Could you check a few things on this model? Use its own coordinates, in mm. A direction names the side the tool comes from. Give positions to 0.01 mm unless a question says otherwise; leave off trailing zeros. Loops run counter-clockwise (first coordinate to the right, second up) from the corner with the lowest first, then second, coordinate; pieces in that order, holes last. Notation, with made-up numbers: M 60,-40 L 83,-40 A17 ccw 83,-13 Z; hole C 69,16 d7. An arc over 180 degrees is marked long. Answer in a Markdown table with one row per item. Add a question column.
```python
from build123d import *

# Parameters (mm, degrees)
SKETCH1_W           = 15
SKETCH1_H           = 21.5
SKETCH1_W_2         = 21.5
SKETCH1_H_2         = 15
BOSS_EXTRUDE1_DEPTH = 1.5
BOSS_EXTRUDE2_START = -1.5
SKETCH2_W           = 1.5
SKETCH2_H           = 15
BOSS_EXTRUDE2_DEPTH = 28.5
BOSS_EXTRUDE3_START = -1.5
SKETCH3_W           = 15
SKETCH3_H           = 1.5
BOSS_EXTRUDE3_DEPTH = 28.5
SKETCH4_R           = 1.5
CUT_EXTRUDE1_DEPTH  = 62
SKETCH5_R           = 1.5
CUT_EXTRUDE2_DEPTH  = 62
FILLET1_R           = 2
FILLET2_R           = 2
FILLET3_R           = 18
CUT_EXTRUDE3_REACH  = 63
SKETCH6_R           = 4
CUT_EXTRUDE4_REACH  = 63
SKETCH7_R           = 4


with BuildPart() as part:
    # Sketch1 → Boss-Extrude1 (new body)
    with BuildSketch(Plane.XY):
        with Locations((0, 18.25)):
            Rectangle(SKETCH1_W, SKETCH1_H)
        with Locations((-18.25, 0)):
            Rectangle(SKETCH1_W_2, SKETCH1_H_2)
        Rectangle(SKETCH1_W, SKETCH1_H_2)
        with Locations((18.25, 0)):
            Rectangle(SKETCH1_W_2, SKETCH1_H_2)
        with Locations((0, -18.25)):
            Rectangle(SKETCH1_W, SKETCH1_H)
    extrude(amount=BOSS_EXTRUDE1_DEPTH)

    # Sketch2 → Boss-Extrude2 (add)
    with BuildSketch(Plane.XY.offset(1.5).offset(BOSS_EXTRUDE2_START)):
        with Locations((-29.75, 0)):
            Rectangle(SKETCH2_W, SKETCH2_H)
        with Locations((29.75, 0)):
            Rectangle(SKETCH2_W, SKETCH2_H)
    extrude(amount=BOSS_EXTRUDE2_DEPTH)

    # Sketch3 → Boss-Extrude3 (add)
    with BuildSketch(Plane(origin=(0, 0, 0), x_dir=(-1, 0, 0), z_dir=(0, 0, -1)).offset(BOSS_EXTRUDE3_START)):
        with Locations((0, 29.75)):
            Rectangle(SKETCH3_W, SKETCH3_H)
        with Locations((0, -29.75)):
            Rectangle(SKETCH3_W, SKETCH3_H)
    extrude(amount=BOSS_EXTRUDE3_DEPTH)

    # Sketch4 → Cut-Extrude1 (cut, through all)
    with BuildSketch(Plane(origin=(30.5, 0, 0), x_dir=(0, 0, -1), z_dir=(1, 0, 0))):
        with Locations((-22.5, 0)):
            Circle(SKETCH4_R)
    extrude(amount=-CUT_EXTRUDE1_DEPTH, mode=Mode.SUBTRACT)

    # Sketch5 → Cut-Extrude2 (cut, through all)
    with BuildSketch(Plane(origin=(0, 30.5, 0), x_dir=(1, 0, 0), z_dir=(0, 1, 0))):
        with Locations((0, 21)):
            Circle(SKETCH5_R)
    extrude(amount=-CUT_EXTRUDE2_DEPTH, mode=Mode.SUBTRACT)

    # Fillet1
    fillet1_edges = [part.edges().sort_by_distance(p)[0] for p in [
        (-7.5, -29.75, -27),
        (7.5, -29.75, -27),
        (-7.5, 29.75, -27),
        (7.5, 29.75, -27),
        (-29.75, 7.5, 28.5),
        (-29.75, -7.5, 28.5),
        (29.75, -7.5, 28.5),
        (29.75, 7.5, 28.5),
    ]]
    fillet(fillet1_edges, radius=FILLET1_R)

    # Fillet2
    fillet2_edges = [part.edges().sort_by_distance(p)[0] for p in [
        (29, 0, 1.5),
        (30.5, 0, 0),
        (-30.5, 0, 0),
        (-29, 0, 1.5),
        (0, 29, 0),
        (0, -29, 0),
        (0, -30.5, 1.5),
        (0, 30.5, 1.5),
    ]]
    fillet(fillet2_edges, radius=FILLET2_R)

    # Fillet3
    fillet3_edges = [part.edges().sort_by_distance(p)[0] for p in [
        (-7.5, 7.5, 0.75),
        (-7.5, -7.5, 0.75),
        (7.5, -7.5, 0.75),
        (7.5, 7.5, 0.75),
    ]]
    fillet(fillet3_edges, radius=FILLET3_R)

    # Sketch6 → Cut-Extrude3 (cut, up to next)
    with BuildSketch(Plane(origin=(30.5, 0, 0), x_dir=(0, 0, -1), z_dir=(1, 0, 0)), mode=Mode.PRIVATE) as cut_extrude3_sk1:
        with Locations((-22.5, 0)):
            Circle(SKETCH6_R)
    cut_extrude3_tool1 = extrude(cut_extrude3_sk1.sketch, amount=-CUT_EXTRUDE3_REACH, mode=Mode.PRIVATE) & part.part
    add(cut_extrude3_tool1.solids().sort_by_distance((30.5, 0, 22.5))[0], mode=Mode.SUBTRACT)

    # Sketch7 → Cut-Extrude4 (cut, up to next)
    with BuildSketch(Plane.XZ.offset(30.5), mode=Mode.PRIVATE) as cut_extrude4_sk1:
        with Locations((0, -21)):
            Circle(SKETCH7_R)
    cut_extrude4_tool1 = extrude(cut_extrude4_sk1.sketch, amount=-CUT_EXTRUDE4_REACH, mode=Mode.PRIVATE) & part.part
    add(cut_extrude4_tool1.solids().sort_by_distance((0, -30.5, -21))[0], mode=Mode.SUBTRACT)


solid = part.part
```
Item 1: If we mould it in two halves opening along Z, with no side actions, what happens to faces 1 (the face through (-30, 0, 24)), 2 (the face through (0.11, -28.4, -0.57)), 3 (the face through (12.633, -12.913, 0.76))? For each: +Z half, -Z half, draft (parallel to the pull), parting line (faces both ways), or undercut.
Item 2: For faces 4 (the face through (-28.4, 0.11, 2.07)), 5 (the face through (0, -29, -14)), 6 (the face through (-12.913, -12.633, 0.76)), which set-ups out of +Z, -Z, +X, -X, +Y, -Y let a thin tool reach every point of the face, with its end or its side?
Item 3: I need wall thicknesses on L1, parallel to Y at x = -30.05, z = 22.5; L2, parallel to Y at x = 29.85, z = 22.5. Which ranges of each line are inside material? Lowest first, please.
Item 4: Suppose I cut it at C-C (z = -21). List the corners of the cut face in (x, y) for me, then the cut area to 3 significant figures.
Item 5: For P1, Ø2.5, axis at y = 0, z = 22.5, coming from the -X side; P2, Ø5, axis at x = -15, y = -4.5, coming from the -Z side; P3, Ø4, axis at x = 29, z = 11, coming from the +Y side; P4, Ø1.5, axis at y = 28.5, z = -8.5, coming from the +X side, each with a flat end and sliding along its axis, tell me the tip position at first contact or that it passes through.
Item 6: Suppose I cut it at D-D (y = -12). List the corners of the cut face in (x, z) for me.
Item 7: Suppose I cut it at B-B (x = 0). List the corners of the cut face in (y, z) for me, then the cut area to 3 significant figures.
Item 8: Suppose I cut it at A-A (z = 17.5). List the corners of the cut face in (x, y) for me, then the cut area to 3 significant figures.
Values found:
| question | item | result |
|---|---|---|
| 1 | face 1 | undercut |
| 1 | face 2 | -Z half |
| 1 | face 3 | draft |
| 2 | face 4 | +Z, +Y, -Y |
| 2 | face 5 | -Z, +X, -X |
| 2 | face 6 | +Z, -Z, -X, -Y |
| 3 | L1 | -7.5 to -1.5, 1.5 to 7.5 |
| 3 | L2 | -7.5 to -4, 4 to 7.5 |
| 4 | outline | M -7.5,-30.5 L -4,-30.5 L -4,-29 L -7.5,-29 Z; M -7.5,29 L -1.5,29 L -1.5,30.5 L -7.5,30.5 Z; M 1.5,29 L 7.5,29 L 7.5,30.5 L 1.5,30.5 Z; M 4,-30.5 L 7.5,-30.5 L 7.5,-29 L 4,-29 Z |
| 4 | area | 28.5 mm² |
| 5 | P1 | through |
| 5 | P2 | z = 0 |
| 5 | P3 | y = 7.5 |
| 5 | P4 | x = 7.5 |
| 6 | outline | M -13.59,0 L 13.59,0 L 13.59,1.5 L -13.59,1.5 Z |
| 7 | outline | M -30.5,-27 L -29,-27 L -29,-25 L -30.5,-25 Z; M -30.5,-17 L -29,-17 L -29,-2 A2 cw -27,0 L 27,0 A2 cw 29,-2 L 29,-19.5 L 30.5,-19.5 L 30.5,-0.5 A2 ccw 28.5,1.5 L -28.5,1.5 A2 ccw -30.5,-0.5 Z; M 29,-27 L 30.5,-27 L 30.5,-22.5 L 29,-22.5 Z |
| 7 | area | 156 mm² |
| 8 | outline | M -30.5,-7.5 L -29,-7.5 L -29,7.5 L -30.5,7.5 Z; M 29,-7.5 L 30.5,-7.5 L 30.5,7.5 L 29,7.5 Z |
| 8 | area | 45.0 mm² |
